Can you work these out from the drawing? Everything is in mm from the part's minimum corner. A direction names the side the tool comes from. Give positions to 0.01 mm unless a question says otherwise; leave off trailing zeros. Order: outer loops, then holes, each group sorted by start corner. A loop starts at its lowest first (then second) coordinate and runs counter-clockwise, first axis right, second up. Notation, with made-up numbers: (-4.75, 15.5) -> (43.25, 15.5) arc R16 ccw to (43.25, 26.5) -> close; hole circle Ø7 at (52.5, 78.25). An arc over 180 degrees is marked (long way). Answer as CSV lines item,"result". Start each with the question number.
(1) Will these pins go through, and if not, where does the flat tip stop? pin 1 Ø17.5 at (x, y) = (26.5, 20) entering from +Z; pin 2 Ø2 at (y, z) = (30.5, 4) entering from +X; pin 3 Ø6.5 at (x, z) = (47, 6) entering from +Y.
(2) I want a section at D-D (z = 11). Please give me the cut outline in (x, y).
(3) I want a section at C-C (y = 20). Please give me the cut outline in (x, z).
(4) We'd pull the mould along X, two halves only. Please class the marked faces 4, 5 and 6: released by +X, released by -X, zero draft, split by the parting line, or undercut.
(5) I want a section at B-B (x = 26.5). Please give me the cut outline in (y, z).
(6) On a 3-axis mill with a long thin cutter (end or side, diameter ignored), from which of +Z, -Z, +X, -X, +Y, -Y can I reach the whole of each face in a straight line? I mean the marked faces 1, 2 and 3. Say none if no direction works.
(7) I want a section at A-A (z = 6). Please give me the cut outline in (x, y), plus the area to 3 significant figures.
(8) I need wall thicknesses on L1, parallel to Z at x = 6, y = 6; L2, parallel to X at y = 20.5, z = 9; L3, parallel to Y at x = 26.5, z = 4.75. Which ranges of each line are inside material? Lowest first, please.
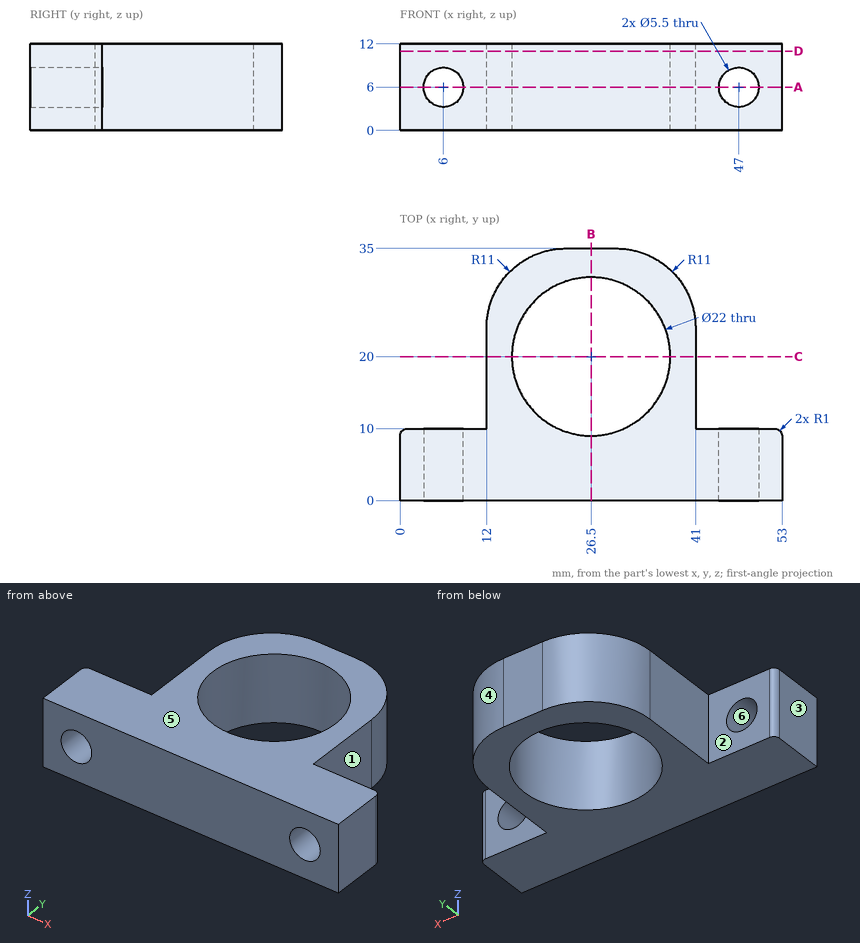
Final values:
1,pin 1,"through"
1,pin 2,"x = 39.53"
1,pin 3,"y = 10"
2,outline,"(0, 0) -> (53, 0) -> (53, 9) arc R1 ccw to (52, 10) -> (41, 10) -> (41, 24) arc R11 ccw to (30, 35) -> (23, 35) arc R11 ccw to (12, 24) -> (12, 10) -> (1, 10) arc R1 ccw to (0, 9) -> close; hole circle Ø22 at (26.5, 20)"
3,outline,"(12, 0) -> (15.5, 0) -> (15.5, 12) -> (12, 12) -> close; (37.5, 0) -> (41, 0) -> (41, 12) -> (37.5, 12) -> close"
4,face 4,"released by +X"
4,face 5,"zero draft"
4,face 6,"undercut"
5,outline,"(0, 0) -> (9, 0) -> (9, 12) -> (0, 12) -> close; (31, 0) -> (35, 0) -> (35, 12) -> (31, 12) -> close"
6,face 1,"+Z, -Z, +X, +Y"
6,face 2,"+Z, -Z, -X, +Y"
6,face 3,"+Z, -Z, -X, +Y, -Y"
7,outline,"(0, 0) -> (3.25, 0) -> (3.25, 10) -> (1, 10) arc R1 ccw to (0, 9) -> close; (8.75, 0) -> (44.25, 0) -> (44.25, 10) -> (41, 10) -> (41, 24) arc R11 ccw to (30, 35) -> (23, 35) arc R11 ccw to (12, 24) -> (12, 10) -> (8.75, 10) -> close; (49.75, 0) -> (53, 0) -> (53, 9) arc R1 ccw to (52, 10) -> (49.75, 10) -> close; hole circle Ø22 at (26.5, 20)"
7,area,"713 mm²"
8,L1,"0 to 3.25, 8.75 to 12"
8,L2,"12 to 15.51, 37.49 to 41"
8,L3,"0 to 9, 31 to 35"
